Check sheet for the drawn part. Datum: minimum x, y, z corner. Units: mm. A direction names the side the tool comes from. Coordinates: 2 decimals unless noted, no trailing zeros. Write each loop counter-clockwise with the first axis right and the second up, starting at its lowest first coordinate (ties: lowest second). Pieces come first, ordered by that corner, then holes. Notation, with made-up numbers: (24.25, 54.25) -> (81.25, 54.25) arc R22 ccw to (81.25, 60.25) -> close; hole circle Ø5 at (5.25, 4.25). An arc over 180 degrees is marked (long way). Answer in a Markdown table with one row per item. Add a question column.
Q1. Section check C-C, the plane z = 17. Record the boundary of the cut face in (x, y).
Q2. Gauge pin test, flat ends, axial feed: P1, Ø1, axis at x = 57.5, z = 10.5, coming from the -Y side; P2, Ø11, axis at x = 147.5, z = 17, coming from the +Y side; P3, Ø1, axis at x = 35.5, y = 15, coming from the -Z side. Record the tip position at first contact, or that the pin passes through.
Q3. Tool access check on the marked faces 1 and 2. Record the directions out of +Z, -Z, +X, -X, +Y, -Y that give a thin tool (end or side, any length) a straight path to the whole face; none if there is none.
Q4. Section check D-D, the plane x = 65. Record the boundary of the cut face in (y, z), and give its area (3 significant figures).
Q5. Thickness scan on line 1 (X direction, y = 59, z = 17); line 2 (Z direction, x = 46.5, y = 45.5); line 3 (Y direction, x = 32, z = 14). Record the ranges inside material, lowest first.
Q6. Release check for a two-part mould opening along Z. For the marked faces 3, 4 and 5 record: pulls with the +Z half, pulls with the -Z half, needs draft (parallel to the pull), parting line crosses it, or undercut.
Q7. Section check B-B, the plane y = 33. Record the boundary of the cut face in (x, z), and give its area (3 significant figures).
Q8. Section check A-A, the plane x = 16. Record the boundary of the cut face in (y, z).
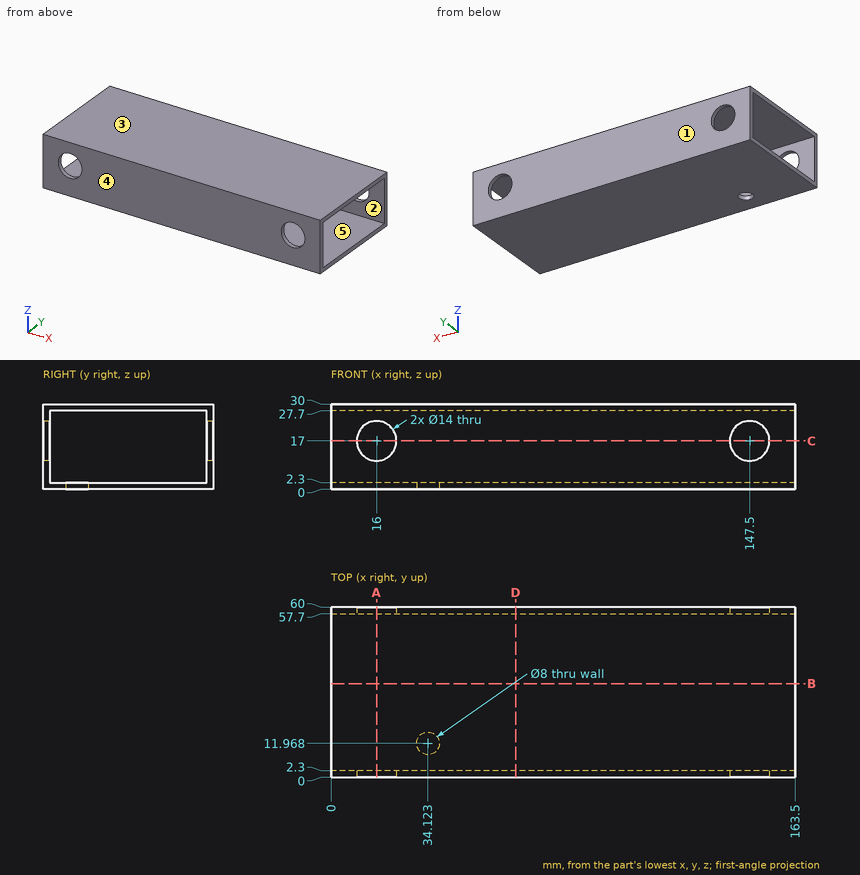
Calculated:
| question | item | result |
|---|---|---|
| 1 | outline | (0, 0) -> (9, 0) -> (9, 2.3) -> (0, 2.3) -> close; (0, 57.7) -> (9, 57.7) -> (9, 60) -> (0, 60) -> close; (23, 0) -> (140.5, 0) -> (140.5, 2.3) -> (23, 2.3) -> close; (23, 57.7) -> (140.5, 57.7) -> (140.5, 60) -> (23, 60) -> close; (154.5, 0) -> (163.5, 0) -> (163.5, 2.3) -> (154.5, 2.3) -> close; (154.5, 57.7) -> (163.5, 57.7) -> (163.5, 60) -> (154.5, 60) -> close |
| 2 | P1 | stops at y = 0 |
| 2 | P2 | passes through |
| 2 | P3 | stops at z = 27.7 |
| 3 | face 1 | +Z, -Z, +X, -X, +Y |
| 3 | face 2 | +X, -X |
| 4 | outline | (0, 0) -> (60, 0) -> (60, 30) -> (0, 30) -> close; hole (2.3, 2.3) -> (57.7, 2.3) -> (57.7, 27.7) -> (2.3, 27.7) -> close |
| 4 | area | 393 mm² |
| 5 | line 1 | x = 0 to 9, 23 to 140.5, 154.5 to 163.5 |
| 5 | line 2 | z = 0 to 2.3, 27.7 to 30 |
| 5 | line 3 | y = 0 to 2.3, 57.7 to 60 |
| 6 | face 3 | pulls with the +Z half |
| 6 | face 4 | needs draft |
| 6 | face 5 | undercut |
| 7 | outline | (0, 0) -> (163.5, 0) -> (163.5, 2.3) -> (0, 2.3) -> close; (0, 27.7) -> (163.5, 27.7) -> (163.5, 30) -> (0, 30) -> close |
| 7 | area | 752 mm² |
| 8 | outline | (0, 0) -> (60, 0) -> (60, 10) -> (57.7, 10) -> (57.7, 2.3) -> (2.3, 2.3) -> (2.3, 10) -> (0, 10) -> close; (0, 24) -> (2.3, 24) -> (2.3, 27.7) -> (57.7, 27.7) -> (57.7, 24) -> (60, 24) -> (60, 30) -> (0, 30) -> close |
